Here's the drawing with two shaded views (mm, measured from the low corner). I have some questions. Round coordinates to 2 decimals unless told otherwise and drop trailing zeros. Loops run counter-clockwise (first coordinate to the right, second up) from the corner with the lowest first, then second, coordinate; pieces in that order, holes last.
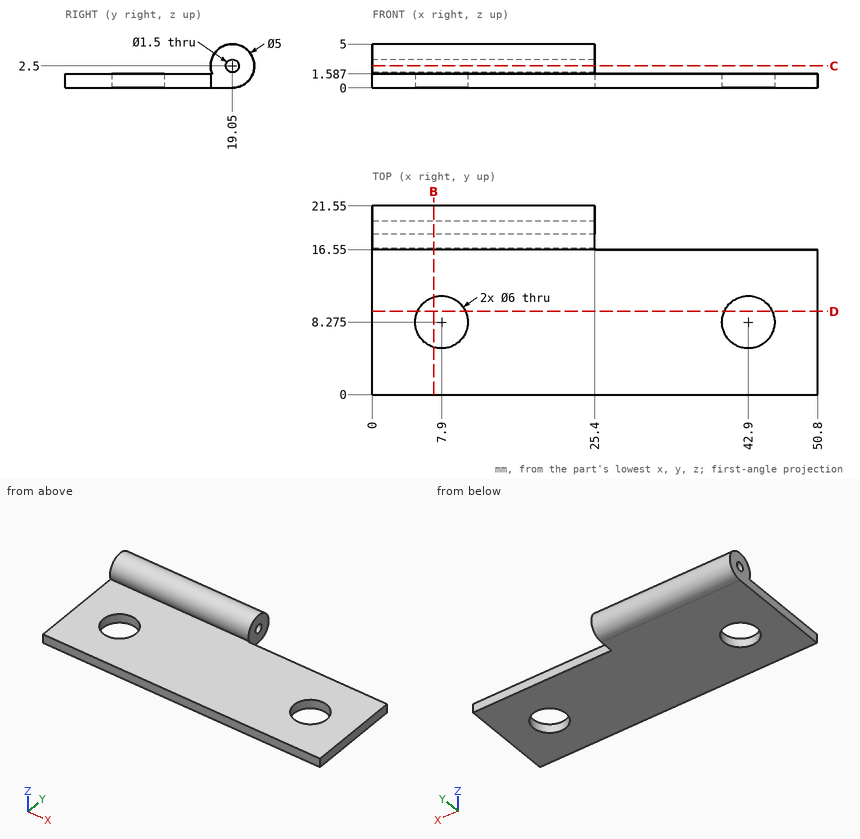
Item 1: If we section it at D-D, the plane y = 9.5: Please give me the cut outline in (x, z).
Results list:
outline: (0, 0) - (5.16, 0) - (5.16, 1.59) - (0, 1.59) - close; (10.64, 0) - (40.16, 0) - (40.16, 1.59) - (10.64, 1.59) - close; (45.64, 0) - (50.8, 0) - (50.8, 1.59) - (45.64, 1.59) - close
Item 2: If I drill on line 1 along Y through (x, z) = (6, 2.5); line 2 along X through (y, z) = (6.5, 0.8); line 3 along Z through (x, y) = (49, 16.5), over which ranges is the centre line in solid material (lowest first)?
Results list:
line 1: y = 16.55 to 18.3, 19.8 to 21.55
line 2: x = 0 to 5.48, 10.32 to 40.48, 45.32 to 50.8
line 3: z = 0 to 1.59
Item 3: Will these pins go through, and if not, where does the flat tip stop? pin 1 (6 mm diameter, centred on x = 45, y = 3.5, fed in from -Z); pin 2 (1.5 mm diameter, centred on y = 15, z = 3.5, fed in from +X); pin 3 (8 mm diameter, centred on x = 42.9, y = 8.275, fed in from +Z); pin 4 (1.7 mm diameter, centred on x = 38.5, z = 0.5, fed in from +Y).
Results list:
pin 1: stops at z = 0
pin 2: passes through
pin 3: stops at z = 1.59
pin 4: stops at y = 16.55
Item 4: If we section it at C-C, the plane z = 2.5: Please give me the cut outline in (x, y).
Results list:
outline: (0, 16.55) - (25.4, 16.55) - (25.4, 18.3) - (0, 18.3) - close; (0, 19.8) - (25.4, 19.8) - (25.4, 21.55) - (0, 21.55) - close
Item 5: If we section it at B-B, the plane x = 7: Please give me the cut outline in (y, z).
Results list:
outline: (0, 0) - (5.41, 0) - (5.41, 1.59) - (0, 1.59) - close; (11.14, 0) - (19.05, 0) arc R2.5 ccw (long way) to (16.72, 1.59) - (11.14, 1.59) - close; hole circle Ø1.5 at (19.05, 2.5)
